```python
from build123d import *

# Parameters (mm, degrees)
SKETCH1_W           = 60
SKETCH1_H           = 10
BOSS_EXTRUDE1_DEPTH = 150
CUT_EXTRUDE1_DEPTH  = 50
FILLET1_R           = 3


with BuildPart() as part:
    # Sketch1 → Boss-Extrude1 (new body)
    with BuildSketch(Plane.XY):
        Rectangle(SKETCH1_W, SKETCH1_H)
    extrude(amount=BOSS_EXTRUDE1_DEPTH)

    # Sketch2 → Cut-Extrude1 (cut)
    with BuildSketch(Plane.XY.offset(150)):
        Polygon((-30, 5), (-30, -5), (0, -5), align=None)
    extrude(amount=-CUT_EXTRUDE1_DEPTH, mode=Mode.SUBTRACT)

    # Fillet1
    fillet1_edges = [part.edges().sort_by_distance(p)[0] for p in [
        (15, -5, 150),
        (-30, -5, 50),
        (-15, -5, 100),
        (30, -5, 75),
    ]]
    fillet(fillet1_edges, radius=FILLET1_R)


solid = part.part
```
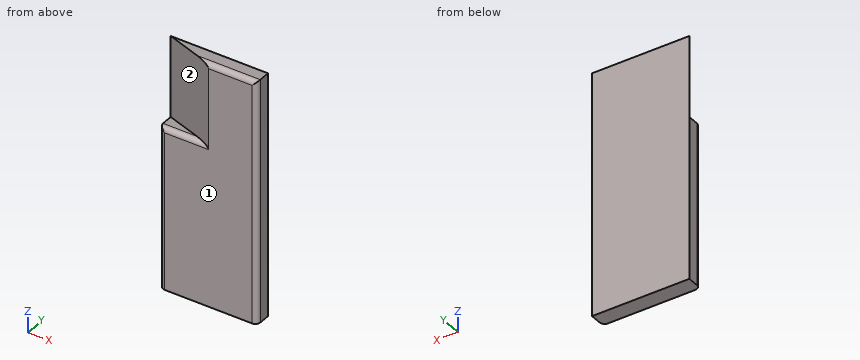
The listing builds one solid part. Answer for the finished solid, in the listing's coordinates (mm). Face numbers are marked on the shaded views. A direction names the side the tool comes from. Round coordinates to 2 decimals unless told otherwise and drop trailing zeros. Write each loop counter-clockwise with the first axis right and the second up, starting at its lowest first coordinate (ties: lowest second). Pieces come first, ordered by that corner, then holes. Notation, with made-up numbers: (8.5, 63) -> (49.5, 63) arc R17 ccw to (49.5, 74) -> close; hole circle Ø4 at (14.5, 43.25). An arc over 180 degrees is marked (long way). Answer as a JSON object with one key per item and string values. Group by question number.
Q1. Each of these flat-tipped pins is pushed along its axis until it touches: pin 1 Ø1.5 at (x, y) = (3, -4) entering from +Z; pin 2 Ø1 at (y, z) = (-3, 112.5) entering from +X. Where does it stop, or does it pass through?
Q2. Straight lines are drawn through the part: line 1 along Z through (x, y) = (-20, 1); line 2 along X through (y, z) = (-2.5, 23.5); line 3 along X through (y, z) = (-4.5, 14). For each, find the intervals that lie inside material, in ascending order.
Q3. Section D-D (x = -17) is taken. Write down the section's boundary in (y, z), plus the area to 3 significant figures.
Q4. Section A-A (y = 3.25) is taken. Write down the section's boundary in (x, z).
Q5. Section C-C (x = -4.5) is taken. Write down the section's boundary in (y, z), plus the area to 3 significant figures.
Q6. Section B-B (z = 108) is taken. Write down the section's boundary in (x, y).
Q7. Which of the six approach directions +Z, -Z, +X, -X, +Y, -Y give full straight-line access (tool end or side, diameter ignored) to the marked faces 1 and 2?
Check values:
{
 "1": {"pin 1": "z = 149.73", "pin 2": "x = 29.96"},
 "2": {"line 1": "0 to 100", "line 2": "-29.96 to 29.96", "line 3": "-28.66 to 28.66"},
 "3": {"outline": "(-5, 0) -> (5, 0) -> (5, 150) -> (0.67, 150) -> (0.67, 100) -> (-2, 100) arc R3 ccw to (-5, 97) -> close", "area": "1,210 mm^2"},
 "4": {"outline": "(-30, 0) -> (30, 0) -> (30, 150) -> (-24.75, 150) -> (-24.75, 100) -> (-30, 100) -> close"},
 "5": {"outline": "(-5, 0) -> (5, 0) -> (5, 150) -> (-2, 150) arc R3 ccw to (-3.5, 149.6) -> (-3.5, 99.6) arc R3 ccw to (-5, 97) -> close", "area": "1,420 mm^2"},
 "6": {"outline": "(-30, 5) -> (0, -5) -> (27, -5) arc R3 ccw to (30, -2) -> (30, 5) -> close"},
 "7": {"face 1": "+Z, -Z, +X, -X, -Y", "face 2": "+Z, -X, -Y"}
}
